Work out the finished part from the listing and answer in its coordinate system (mm). A direction names the side the tool comes from. Round coordinates to 2 decimals unless told otherwise and drop trailing zeros. Return JSON: item names as keys, results as strings.
from build123d import *

# Parameters (mm, degrees)
SKETCH1_W           = 45
SKETCH1_H           = 45
BOSS_EXTRUDE1_DEPTH = 45
CUT_EXTRUDE1_DEPTH  = 3
FILLET1_R           = 2
BOSS_EXTRUDE2_DEPTH = 3
FILLET2_R           = 2
FILLET3_R           = 2


with BuildPart() as part:
    # Sketch1 → Boss-Extrude1 (new body)
    with BuildSketch(Plane(origin=(0, 0, 0), x_dir=(1, 0, 0), z_dir=(0, 1, 0))):
        with Locations((22.5, 22.5)):
            Rectangle(SKETCH1_W, SKETCH1_H)
    extrude(amount=BOSS_EXTRUDE1_DEPTH)

    # Sketch2 → Cut-Extrude1 (cut)
    with BuildSketch(Plane(origin=(0, 45, 0), x_dir=(1, 0, 0), z_dir=(0, 1, 0))):
        with BuildLine():
            Line((6, 41), (39, 41))
            ThreePointArc((39, 41), (40.414213562, 40.414213562), (41, 39))
            Line((41, 39), (41, 6))
            ThreePointArc((41, 6), (40.414213562, 4.585786438), (39, 4))
            Line((39, 4), (6, 4))
            ThreePointArc((6, 4), (4.585786438, 4.585786438), (4, 6))
            Line((4, 6), (4, 39))
            ThreePointArc((4, 39), (4.585786438, 40.414213562), (6, 41))
        make_face()
    extrude(amount=-CUT_EXTRUDE1_DEPTH, mode=Mode.SUBTRACT)

    # Fillet1
    fillet1_edges = [part.edges().sort_by_distance(p)[0] for p in [
        (40.414213562, 42, -40.414213562),
        (41, 42, -22.5),
        (40.414213562, 42, -4.585786438),
        (22.5, 42, -4),
        (4.585786438, 42, -4.585786438),
        (4, 42, -22.5),
        (4.585786438, 42, -40.414213562),
        (22.5, 42, -41),
    ]]
    fillet(fillet1_edges, radius=FILLET1_R)

    # Sketch3 → Boss-Extrude2 (add)
    with BuildSketch(Plane(origin=(0, 42, 0), x_dir=(1, 0, 0), z_dir=(0, 1, 0))):
        with BuildLine():
            Line((38.242693353, 9.243196233), (23.656388738, 9.243196233))
            Line((23.656388738, 9.243196233), (23.656388738, 10.666250342))
            add(Edge.make_bspline(
                [(23.656388738, 10.666250342), (23.840076099, 10.68078989), (24.225242332, 10.711277253), (24.822230957, 10.802993535), (25.469379926, 10.895689338), (26.022940834, 11.010248275), (26.463008214, 11.096809674), (26.751861609, 11.185019051), (27.001950694, 11.262002653), (27.202632415, 11.353541525), (27.365753511, 11.438699124), (27.476844631, 11.539421658), (27.55548257, 11.642841951), (27.565194032, 11.719511547), (27.569787537, 11.755776144)],
                knots=[0, 0, 0, 0, 1.580663375, 3.314425972, 5.180984338, 7.189265601, 8.165445891, 9.025996966, 9.780234646, 10.406650621, 10.91943364, 11.347278432, 11.691263739, 12, 12, 12, 12], degree=3))
            add(Edge.make_bspline(
                [(27.569787537, 11.755776144), (27.569435107, 11.809650716), (27.568689302, 11.923658657), (27.533827132, 12.110664377), (27.487076537, 12.345104426), (27.419571412, 12.510976182), (27.380788164, 12.606273326)],
                knots=[0, 0, 0, 0, 0.735694078, 1.556856296, 2.596357679, 4, 4, 4, 4], degree=3))
            Line((27.380788164, 12.606273326), (25.073884042, 18.137284413))
            Line((25.073884042, 18.137284413), (15.618356546, 18.137284413))
            add(Edge.make_bspline(
                [(15.618356546, 18.137284413), (15.504836551, 17.857690943), (15.261095281, 17.257369675), (14.897005839, 16.330696191), (14.552517174, 15.390865424), (14.332060663, 14.774334183), (14.228655267, 14.485149454)],
                knots=[0, 0, 0, 0, 0.926583958, 1.989488725, 3.056967239, 4, 4, 4, 4], degree=3))
            add(Edge.make_bspline(
                [(14.228655267, 14.485149454), (14.174323811, 14.322282922), (14.073992132, 14.021523953), (13.944497555, 13.605517058), (13.852124744, 13.261079178), (13.790356149, 12.921159244), (13.757506332, 12.61062748), (13.744527557, 12.391364177), (13.739480418, 12.30609785)],
                knots=[0, 0, 0, 0, 1.377792625, 2.544313332, 3.496463908, 4.237287142, 5.314522549, 6, 6, 6, 6], degree=3))
            add(Edge.make_bspline(
                [(13.739480418, 12.30609785), (13.752275343, 12.20703328), (13.779291631, 11.997859957), (13.987544963, 11.717644303), (14.302946626, 11.47080153), (14.743758449, 11.250468253), (15.325360636, 11.057952059), (16.061834345, 10.898701284), (16.958602595, 10.761686661), (17.611688564, 10.699703767), (17.964172303, 10.666250342)],
                knots=[0, 0, 0, 0, 0.491092674, 1.036934666, 1.680532576, 2.482252872, 3.47863382, 4.729366136, 6.234772593, 8, 8, 8, 8], degree=3))
            Line((17.964172303, 10.666250342), (17.964172303, 9.243196233))
            Line((17.964172303, 9.243196233), (6.93550296, 9.243196233))
            Line((6.93550296, 9.243196233), (6.93550296, 10.666250342))
            add(Edge.make_bspline(
                [(6.93550296, 10.666250342), (7.156458841, 10.68507928), (7.626766221, 10.725156912), (8.214255419, 10.83449568), (8.694916504, 10.934535131), (9.021428402, 11.044189086), (9.31379367, 11.154502307), (9.484333571, 11.253318866), (9.564817778, 11.299954125)],
                knots=[0, 0, 0, 0, 1.463204883, 3.114450051, 3.942471061, 4.700769028, 5.386843935, 6, 6, 6, 6], degree=3))
            add(Edge.make_bspline(
                [(9.564817778, 11.299954125), (9.808806898, 11.456132653), (10.289617679, 11.763901787), (10.894760398, 12.38121249), (11.401516748, 13.103822817), (11.641967893, 13.651883003), (11.766104603, 13.934827748)],
                knots=[0, 0, 0, 0, 0.990620078, 1.952139562, 2.94275964, 4, 4, 4, 4], degree=3))
            add(Edge.make_bspline(
                [(11.766104603, 13.934827748), (12.49384773, 15.674926569), (13.950269602, 19.157361354), (15.787937069, 23.531851641), (17.281093989, 27.110474834), (18.468273477, 29.928542487), (19.704638443, 32.883483751), (20.55061589, 34.89718826), (20.982603479, 35.925460773)],
                knots=[0, 0, 0, 0, 1.423871405, 2.8495734, 3.581899029, 4.351134106, 5.15802767, 6, 6, 6, 6], degree=3))
            Line((20.982603479, 35.925460773), (24.740355735, 35.925460773))
            add(Edge.make_bspline(
                [(24.740355735, 35.925460773), (25.037951878, 35.198811204), (25.616719472, 33.785616739), (26.473021768, 31.729065196), (27.262884583, 29.784355708), (28.012276259, 27.959201793), (28.701657163, 26.247813786), (29.358282986, 24.658333454), (29.948553903, 23.180808533), (30.499990304, 21.811943928), (31.011657569, 20.529416983), (31.511007395, 19.316516594), (31.980152709, 18.154453259), (32.436507788, 17.051074697), (32.870912199, 16.001880065), (33.286642483, 15.010835315), (33.682273223, 14.072862205), (33.941746737, 13.467767085), (34.068030714, 13.173271448)],
                knots=[0, 0, 0, 0, 1.532752056, 2.980909665, 4.348409991, 5.629937521, 6.832191988, 7.949838466, 8.98685575, 9.937901843, 10.830515139, 11.682178711, 12.498237346, 13.276712205, 14.012891946, 14.714850756, 15.374526692, 16, 16, 16, 16], degree=3))
            add(Edge.make_bspline(
                [(34.068030714, 13.173271448), (34.156473839, 12.994922089), (34.332453747, 12.640051048), (34.679517564, 12.137203398), (35.154116348, 11.674345926), (35.54643409, 11.431082086), (35.757907468, 11.299954125)],
                knots=[0, 0, 0, 0, 0.929211814, 1.848901312, 2.840480417, 4, 4, 4, 4], degree=3))
            add(Edge.make_bspline(
                [(35.757907468, 11.299954125), (35.94634352, 11.206794224), (36.337568372, 11.013378643), (36.978994102, 10.838934171), (37.620953448, 10.729278261), (38.044146103, 10.686377762), (38.242693353, 10.666250342)],
                knots=[0, 0, 0, 0, 0.974847381, 2.023946679, 3.072904627, 4, 4, 4, 4], degree=3))
            Line((38.242693353, 10.666250342), (38.242693353, 9.243196233))
        make_face()
        Polygon((24.317886547, 19.916102049), (20.315546866, 29.799657539), (16.357677626, 19.916102049), align=None, mode=Mode.SUBTRACT)
    extrude(amount=BOSS_EXTRUDE2_DEPTH)

    # Fillet2
    fillet2_edges = [part.edges().sort_by_distance(p)[0] for p in [
        (45, 22.5, -45),
        (45, 22.5, 0),
        (0, 22.5, 0),
    ]]
    fillet(fillet2_edges, radius=FILLET2_R)

    # Fillet3
    fillet3_edges = [part.edges().sort_by_distance(p)[0] for p in [
        (0, 22.5, -45),
    ]]
    fillet(fillet3_edges, radius=FILLET3_R)


solid = part.part
1) Find the intervals of material crossed by L1, parallel to X at y = 43, z = -16; L2, parallel to Y at x = 16, z = -12; L3, parallel to Y at x = 8.5, z = -5, in increasing order.
Verdict:
{"L1": "x = 0 to 4.27, 12.63 to 14.78, 25.97 to 32.87, 40.73 to 45", "L2": "y = 0 to 42", "L3": "y = 0 to 42.27"}
2) Flat-ended cylindrical pins translate along their axes: pin 1 (9 mm diameter, centred on x = 22, z = -24, fed in from +Y); pin 2 (2 mm diameter, centred on x = 12, z = -39, fed in from +Y). Find the tip coordinate at first contact, or state that the pin passes through.
Verdict:
{"pin 1": "stops at y = 45", "pin 2": "stops at y = 42.27"}
3) A tool of negligible diameter and unlimited length cuts with its end or side. For faces 1 (the flat face through (45, 22, -22)), 2 (the flat face through (22.345, 43.479, -24.789)), from which of +Z, -Z, +X, -X, +Y, -Y can it reach the whole face along a straight path? Write none if from no direction.
Verdict:
{"face 1": "+Z, -Z, +X, +Y, -Y", "face 2": "+Y"}
4) Determine the mould class of faces 3 (the cylindrical face through (44.4, 22.82, -0.57)), 4 (the flat face through (22, 22, 0)), 5 (the cylindrical face through (4.57, 44.51, -40.4)) for opening direction X: pulls with the +X half, pulls with the -X half, needs draft (parallel to the pull), parting line crosses it, or undercut.
Verdict:
{"face 3": "pulls with the +X half", "face 4": "needs draft", "face 5": "undercut"}
